```python
from build123d import *

# Parameters (mm, degrees)
SKETCH_1_W             = 160
SKETCH_1_H             = 44.5
EXTRUDE_1_DEPTH        = 28.7
FILLET_1_R             = 5
CHAMFER_1_SIZE         = 30
CHAMFER_1_SIZE2        = 4.75153321
CHAMFER_1_PART_2_SIZE  = 30
CHAMFER_1_PART_2_SIZE2 = 4.75153321
EXTRUDE_6_DEPTH        = 120
EXTRUDE_7_DEPTH        = 50
SKETCH_3_R             = 1.75
EXTRUDE_8_DEPTH        = 7.5
SKETCH_3_3_R           = 1.75
EXTRUDE_9_DEPTH        = 16
SKETCH_4_R             = 1.75
CUT_EXTRUDE_1_DEPTH    = 8


with BuildPart() as part:
    # Sketch 1 → Extrude 1 (new body)
    with BuildSketch(Plane.XY):
        with Locations((80, 22.25)):
            Rectangle(SKETCH_1_W, SKETCH_1_H)
    extrude(amount=EXTRUDE_1_DEPTH)

    # Fillet 1
    fillet_1_edges = [part.edges().sort_by_distance(p)[0] for p in [
        (160, 22.25, 28.7),
        (160, 22.25, 0),
    ]]
    fillet(fillet_1_edges, radius=FILLET_1_R)

    # Chamfer 1
    chamfer_1_edges = [part.edges().sort_by_distance(p)[0] for p in [
        (0, 22.25, 28.7),
    ]]
    chamfer_1_side = [part.faces().sort_by_distance(p)[0] for p in [
        (77.5, 22.25, 28.7),
    ]]
    chamfer(chamfer_1_edges, length=CHAMFER_1_SIZE, length2=CHAMFER_1_SIZE2, reference=chamfer_1_side[0])

    # Chamfer 1 part 2
    chamfer_1_part_2_edges = [part.edges().sort_by_distance(p)[0] for p in [
        (0, 22.25, 0),
    ]]
    chamfer_1_part_2_side = [part.faces().sort_by_distance(p)[0] for p in [
        (77.5, 22.25, 0),
    ]]
    chamfer(chamfer_1_part_2_edges, length=CHAMFER_1_PART_2_SIZE, length2=CHAMFER_1_PART_2_SIZE2, reference=chamfer_1_part_2_side[0])

    # Sketch 2 → Extrude 6 (add)
    with BuildSketch(Plane.ZY):
        with BuildLine():
            Line((16.475, 44.5), (12.225, 44.5))
            ThreePointArc((12.225, 44.5), (10.1, 42.375), (12.225, 40.25))
            Line((12.225, 40.25), (16.474999883, 40.25))
            ThreePointArc((16.474999883, 40.25), (18.6, 42.374999942), (16.475, 44.5))
        make_face()
    extrude(amount=EXTRUDE_6_DEPTH)

    # Sketch 2_3 → Extrude 7 (add)
    with BuildSketch(Plane.ZY):
        with BuildLine():
            ThreePointArc((11.35, 2), (10.35, 1), (11.35, 0))
            Line((11.35, 0), (17.35, 0))
            ThreePointArc((17.35, 0), (18.35, 1), (17.35, 2))
            Line((17.35, 2), (11.35, 2))
        make_face()
    extrude(amount=EXTRUDE_7_DEPTH)

    # Sketch 3 → Extrude 8 (add)
    with BuildSketch(Plane.ZY.offset(104)):
        Polygon((6.35, 43.875), (6.35, 40.875), (8.85, 38.375), (22.35, 38.375), (22.35, 46.375), (8.85, 46.375), align=None)
        Polygon((14.746028023, 39.175), (21.35, 39.175), (21.35, 45.575), (9.85, 45.575), (7.35, 43.075), (7.35, 41.675), (9.85, 39.175), (14.11665296, 39.175), (14.11665296, 40.489122918), (14.746028023, 40.489122918), align=None, mode=Mode.SUBTRACT)
        Polygon((14.746028023, 39.175), (14.746028023, 40.489122918), (14.11665296, 40.489122918), (14.11665296, 39.175), (9.85, 39.175), (7.35, 41.675), (7.35, 43.075), (9.85, 45.575), (21.35, 45.575), (21.35, 39.175), align=None)
        with Locations((12.225, 42.375)):
            Circle(SKETCH_3_R, mode=Mode.SUBTRACT)
        with Locations((16.475, 42.375)):
            Circle(SKETCH_3_R, mode=Mode.SUBTRACT)
        with Locations((12.225, 42.375)):
            Circle(SKETCH_3_R)
        with Locations((16.475, 42.375)):
            Circle(SKETCH_3_R)
    extrude(amount=EXTRUDE_8_DEPTH)

    # Sketch 3_3 → Extrude 9 (add)
    with BuildSketch(Plane.ZY.offset(104)):
        Polygon((14.746028023, 39.175), (14.746028023, 40.489122918), (14.11665296, 40.489122918), (14.11665296, 39.175), (9.85, 39.175), (7.35, 41.675), (7.35, 43.075), (9.85, 45.575), (21.35, 45.575), (21.35, 39.175), align=None)
        with Locations((12.225, 42.375)):
            Circle(SKETCH_3_3_R, mode=Mode.SUBTRACT)
        with Locations((16.475, 42.375)):
            Circle(SKETCH_3_3_R, mode=Mode.SUBTRACT)
    extrude(amount=EXTRUDE_9_DEPTH)

    # Sketch 4 → Cut-Extrude 1 (cut)
    with BuildSketch(Plane.ZY.offset(120)):
        with Locations((11.633674327, 42.375)):
            Circle(SKETCH_4_R)
        with Locations((17.123250996, 42.375)):
            Circle(SKETCH_4_R)
    extrude(amount=-CUT_EXTRUDE_1_DEPTH, mode=Mode.SUBTRACT)


solid = part.part
```
Source: CAD feature listing. Evaluate the final solid. Frame: model axes, mm. A direction names the side the tool comes from. Coordinates: 2 decimals unless noted, no trailing zeros. Loops run counter-clockwise (first coordinate to the right, second up) from the corner with the lowest first, then second, coordinate; pieces in that order, holes last. Notation, with made-up numbers: (-33.75, -10.5) -> (17.25, -10.5) arc R6 cw to (17.25, -1.5) -> close; hole circle Ø5 at (-4.75, -1.75). An arc over 180 degrees is marked (long way). One line per item, written item: value. Start each with the question number.
Q1. Line query: line 1 along X through (y, z) = (42.5, 8.75); line 2 along X through (y, z) = (38.5, 19.75); line 3 along X through (y, z) = (21, 7.5). Output: solid intervals per line, ascending.
Q2. Mould query, pull axis Y, two halves, no side actions, for faces 6 (the face through (-108, 46.375, 16)), 7 (the face through (0, 22, 14)), 8 (the face through (-111.5, 39, 14)). Classes: pulls with the +Y half, pulls with the -Y half, needs draft (parallel to the pull), parting line crosses it, or undercut.
Q3. Contact query for flat-ended pins moving along their axis: P1, Ø2, axis at x = -68, z = 14.5, coming from the -Y side; P2, Ø4, axis at x = -0.5, y = 22, coming from the -Z side; P3, Ø2, axis at x = 46, z = 16.5, coming from the +Y side. Output: stop coordinate, or through.
Q4. Section query A-A, the plane x = -16. Return the cut outline in (y, z) (3 decimals).
Q5. Section query C-C, the plane x = 33. Return the cut outline in (y, z).
Q6. Section query B-B, the plane y = 26. Return the cut outline in (x, z).
Q7. Set-up query: faces 1 (the face through (-104, 40, 14)), 2 (the face through (85, 44.5, 14)), 3 (the face through (-116, 45.575, 16)), 4 (the face through (-116, 42, 21.35)), 5 (the face through (-116, 39.175, 18)). Return all of +Z, -Z, +X, -X, +Y, -Y with unobstructed straight access to the full face (end or side cutting, diameter ignored); none if empty.
Results:
1. line 1: -120 to -104, 0 to 160
1. line 2: -111.5 to -104, 0 to 160
1. line 3: 0 to 160
2. face 6: pulls with the +Y half
2. face 7: undercut
2. face 8: needs draft
3. P1: y = 40.25
3. P2: z = 4.51
3. P3: y = 44.5
4. outline: (0, 11.35) arc R1 ccw to (2, 11.35) -> (2, 17.35) arc R1 ccw to (0, 17.35) -> close; (40.25, 12.225) arc R2.125 ccw to (44.5, 12.225) -> (44.5, 16.475) arc R2.125 ccw to (40.25, 16.475) -> close
5. outline: (0, 0) -> (44.5, 0) -> (44.5, 28.7) -> (0, 28.7) -> close
6. outline: (0, 4.75) -> (30, 0) -> (155, 0) arc R5 ccw to (160, 5) -> (160, 23.7) arc R5 ccw to (155, 28.7) -> (30, 28.7) -> (0, 23.95) -> close
7. face 1: none
7. face 2: +Z, -Z, +X, +Y
7. face 3: +Z, -Z, -X, +Y
7. face 4: +Z, -X, +Y, -Y
7. face 5: +Z, -Z, -X, -Y
